```python
from build123d import *

# Parameters (mm, degrees)
F0_W     = 50.8
F0_H     = 19.5178945826
F0_H_2   = 14.4378958169
F0_W_2   = 18.715784845
F0_W_3   = 8.0210510887
F0_H_3   = 2.1389448998
F0_H_4   = 12.0315781759
F0_H_5   = 22.9936808162
F0_H_6   = 0.5347377678
F1_DEPTH = 25.4
F3_DEPTH = 25.4
F4_W     = 50.4511781037
F4_H     = 18.8805037178
F5_DEPTH = 34.798


with BuildPart() as f1:
    # F0 (on Front) → F1 (new body)
    with BuildSketch(Plane.XZ):
        with Locations((0.4468671068, 36.4022840108)):
            Rectangle(F0_W, F0_H)
        with Locations((0.4468671068, 19.4243888111)):
            Rectangle(F0_W, F0_H_2)
        Polygon((-24.9531328932, 12.2054409026), (-24.9531328932, 26.6433367195), (-42.332081033, 26.6433367195), (-42.332081033, 12.2054409026), (-46.0752392364, 12.2054409026), (-46.0752392364, -19.3440310844), (-42.332081033, -19.3440310844), (-42.332081033, -31.3756092603), (-24.9531328932, -31.3756092603), (-24.9531328932, -19.3440310844), (25.8468671068, -19.3440310844), (44.5626519519, -19.3440310844), (52.5837030406, -19.3440310844), (56.3268581581, -19.3440310844), (56.3268581581, 12.2054409026), (52.5837030406, 12.2054409026), (44.5626519519, 12.2054409026), (25.8468671068, 12.2054409026), align=None)
        with Locations((35.2047595293, 19.4243888111)):
            Rectangle(F0_W_2, F0_H_2)
        with Locations((48.5731774962, 19.4243888111)):
            Rectangle(F0_W_3, F0_H_2)
        with Locations((48.5731774962, 27.7128091694)):
            Rectangle(F0_W_3, F0_H_3)
        Polygon((84.667918967, 26.6433367195), (52.5837030406, 26.6433367195), (52.5837030406, 12.2054409026), (56.3268581581, 12.2054409026), (84.667918967, 12.2054409026), align=None)
        Polygon((84.667918967, -19.3440310844), (56.3268581581, -19.3440310844), (52.5837030406, -19.3440310844), (52.5837030406, -31.3756092603), (84.667918967, -31.3756092603), align=None)
        with Locations((48.5731774962, -25.3598201724)):
            Rectangle(F0_W_3, F0_H_4)
        with Locations((0.4468671068, -25.3598201724)):
            Rectangle(F0_W, F0_H_4)
        with Locations((0.4468671068, -42.8724496684)):
            Rectangle(F0_W, F0_H_5)
        with Locations((35.2047595293, -25.3598201724)):
            Rectangle(F0_W_2, F0_H_4)
        with Locations((48.5731774962, -31.6429781442)):
            Rectangle(F0_W_3, F0_H_6)
    extrude(amount=F1_DEPTH)

    # F2 (on face) → F3 (join)
    with BuildSketch(Plane.XZ.offset(25.4)):
        Polygon((8.8767074049, 26.6433367195), (-9.6942791715, 26.6433367195), (-9.6942791715, 19.0352611244), (-24.9531328932, 19.0352611244), (-24.9531328932, 11.2973507494), (-37.8602743149, 11.2973507494), (-37.8602743149, -12.8449322656), (-24.9531328932, -12.8449322656), (-24.9531328932, -20.2733278275), (-9.6942791715, -20.2733278275), (-9.6942791715, -33.8920503855), (8.8767074049, -33.8920503855), (8.8767074049, -27.701722458), (77.8988748789, -27.701722458), (77.8988748789, -23.3684927225), (48.8043278456, -23.3684927225), (48.8043278456, 16.5591295809), (76.6608119011, 16.5591295809), (76.6608119011, 22.1304260194), (8.8767074049, 22.1304260194), align=None)
    extrude(amount=F3_DEPTH)

    # F4 (on face) → F5 (join)
    with BuildSketch(Plane.XZ.offset(50.8)):
        with Locations((8.1029143184, -2.7856479865)):
            Rectangle(F4_W, F4_H)
    extrude(amount=F5_DEPTH)


solid = f1.part
```
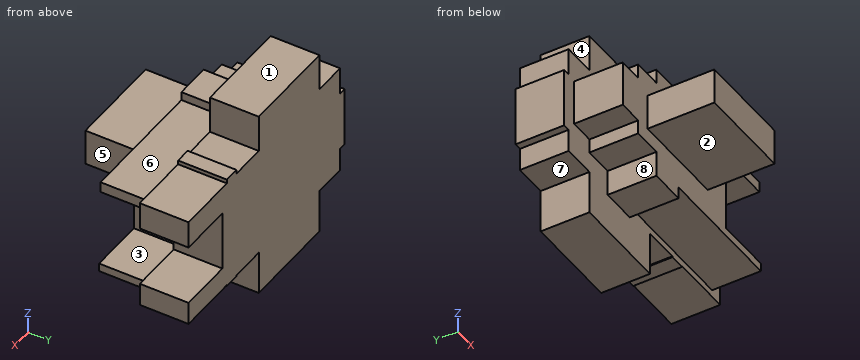
Geometry check sheet. Reference: the model listing, model coordinates, mm. Face numbers are marked on the shaded views. A direction names the side the tool comes from. Give positions to 0.01 mm unless a question says otherwise; leave off trailing zeros. Write each loop counter-clockwise with the first axis right and the second up, starting at its lowest first coordinate (ties: lowest second). Pieces come first, ordered by that corner, then holes. Notation, with made-up numbers: (-19, -12.5) -> (23, -12.5) arc R12 ccw to (23, 0.5) -> close; hole circle Ø1 at (21, 32.5). An arc over 180 degrees is marked (long way). Use one line per item in the form item = value.
Item 1: Scan lines: line 1 (Z direction, x = 56.5, y = -39); line 2 (X direction, y = -20.5, z = 27.5); line 3 (Y direction, x = -9.5, z = -27). Record each from-to range of solid material in increasing order.
Results list:
line_1 = -27.7 to -23.37, 16.56 to 22.13
line_2 = -24.95 to 25.85, 44.56 to 52.58
line_3 = -50.8 to 0
Item 2: Depth check by flat-ended pin: pin 1 Ø3 at (y, z) = (-13.5, 29) entering from -X; pin 2 Ø12 at (x, y) = (-11, -59.5) entering from -Z; pin 3 Ø10 at (y, z) = (-39.5, -32) entering from +X; pin 4 Ø20.5 at (x, y) = (32.5, -7.5) entering from -Z. Enter the tip coordinate at first touch or a pass-through.
Results list:
pin_1 = -24.95
pin_2 = -12.23
pin_3 = 77.9
pin_4 = -54.37
Item 3: Mould release check, pull along Z, two halves, no side actions. Record for the marked faces 1, 2 and 3: released by +Z, released by -Z, zero draft, split by the parting line, or undercut.
Results list:
face_1 = released by +Z
face_2 = released by -Z
face_3 = undercut
Item 4: Sectioned sample at C-C on y = -47. Enter the section's corners in (x, z).
Results list:
outline = (-37.86, -12.84) -> (-24.95, -12.84) -> (-24.95, -20.27) -> (-9.69, -20.27) -> (-9.69, -33.89) -> (8.88, -33.89) -> (8.88, -27.7) -> (77.9, -27.7) -> (77.9, -23.37) -> (48.8, -23.37) -> (48.8, 16.56) -> (76.66, 16.56) -> (76.66, 22.13) -> (8.88, 22.13) -> (8.88, 26.64) -> (-9.69, 26.64) -> (-9.69, 19.04) -> (-24.95, 19.04) -> (-24.95, 11.3) -> (-37.86, 11.3) -> close
Item 5: Sectioned sample at B-B on z = -16. Enter the section's corners in (x, y).
Results list:
outline = (-46.08, -25.4) -> (-24.95, -25.4) -> (-24.95, -50.8) -> (48.8, -50.8) -> (48.8, -25.4) -> (56.33, -25.4) -> (56.33, 0) -> (-46.08, 0) -> close
Item 6: Sectioned sample at D-D on x = -14. Enter the section's corners in (y, z).
Results list:
outline = (-85.6, -12.23) -> (-50.8, -12.23) -> (-50.8, -20.27) -> (-25.4, -20.27) -> (-25.4, -54.37) -> (0, -54.37) -> (0, 46.16) -> (-25.4, 46.16) -> (-25.4, 19.04) -> (-50.8, 19.04) -> (-50.8, 6.65) -> (-85.6, 6.65) -> close
Item 7: Access from +Z, -Z, +X, -X, +Y, -Y to the whole of each face (thin tool, end or side, straight path). Record for the marked faces 4, 5, 6, 7 and 8.
Results list:
face_4 = +Z, -X, +Y, -Y
face_5 = +Z, -Z, +X, -Y
face_6 = +Z, +X, -Y
face_7 = -Z, -X, +Y, -Y
face_8 = -Z, -X, -Y
Item 8: Sectioned sample at A-A on x = 69. Enter the section's corners in (y, z), plus the area to 3 significant figures.
Results list:
outline = (-50.8, -27.7) -> (-25.4, -27.7) -> (-25.4, -31.38) -> (0, -31.38) -> (0, -19.34) -> (-25.4, -19.34) -> (-25.4, -23.37) -> (-50.8, -23.37) -> close; (-50.8, 16.56) -> (-25.4, 16.56) -> (-25.4, 12.21) -> (0, 12.21) -> (0, 26.64) -> (-25.4, 26.64) -> (-25.4, 22.13) -> (-50.8, 22.13) -> close
area = 924 mm2
